from build123d import *

# Parameters (mm, degrees)
SKETCH1_R           = 1.524
BOSS_EXTRUDE1_DEPTH = 6.35


with BuildPart() as part:
    # Sketch1 → Boss-Extrude1 (new body)
    with BuildSketch(Plane(origin=(0, 0, 0), x_dir=(1, 0, 0), z_dir=(0, 1, 0))):
        with BuildLine():
            Line((23.368, 0), (17.018, 0))
            Line((17.018, 0), (17.018, 5.534999979))
            Line((17.018, 5.534999979), (19.058999982, 5.534999979))
            Line((19.058999982, 5.534999979), (19.058999982, 8.435000021))
            Line((19.058999982, 8.435000021), (17.018, 8.435000021))
            Line((17.018, 8.435000021), (17.018, 13.97))
            Line((17.018, 13.97), (12.7, 13.97))
            Line((12.7, 13.97), (12.7, 8.435000021))
            Line((12.7, 8.435000021), (10.659000018, 8.435000021))
            Line((10.659000018, 8.435000021), (10.659000018, 5.534999979))
            Line((10.659000018, 5.534999979), (12.7, 5.534999979))
            Line((12.7, 5.534999979), (12.7, 0))
            Line((12.7, 0), (6.35, 0))
            Line((6.35, 0), (6.35, -6.35))
            Line((6.35, -6.35), (0, -6.35))
            Line((0, -6.35), (0, 0))
            Line((0, 0), (-15.24, 22.286579861))
            ThreePointArc((-15.24, 22.286579861), (-12.038790491, 39.334629649), (5.009259297, 36.133420139))
            Line((5.009259297, 36.133420139), (29.718, 0))
            Line((29.718, 0), (29.718, -6.35))
            Line((29.718, -6.35), (23.368, -6.35))
            Line((23.368, -6.35), (23.368, 0))
        make_face()
        with Locations(Location((-5.115370351, 29.21, 0), (0, 0, 270))):
            Circle(SKETCH1_R, mode=Mode.SUBTRACT)
    extrude(amount=BOSS_EXTRUDE1_DEPTH)


solid = part.part
Verification items for the finished model (mm, model axes). A direction names the side the tool comes from. Round coordinates to 2 decimals unless told otherwise and drop trailing zeros. Loops run counter-clockwise (first coordinate to the right, second up) from the corner with the lowest first, then second, coordinate; pieces in that order, holes last. Notation, with made-up numbers: (80.25, -31.75) - (106.25, -31.75) arc R13 cw to (106.25, -14.75) - close; hole circle Ø11 at (66.25, 17.5). An arc over 180 degrees is marked (long way). Answer in a Markdown table with one row per item. Add a question column.
Q1. Tool access check on faces 1 (the face through (27, 3, 6.35)), 2 (the face through (12, 3, -8.435)), 3 (the face through (15, 3, -13.97)). Record the directions out of +Z, -Z, +X, -X, +Y, -Y that give a thin tool (end or side, any length) a straight path to the whole face; none if there is none.
Q2. Release check for a two-part mould opening along X. For faces 4 (the face through (10, 3, 0)), 5 (the face through (29.718, 3, 3)), 6 (the face through (0, 3, 3)), 7 (the face through (12.7, 3, -11)) record: pulls with the +X half, pulls with the -X half, needs draft (parallel to the pull), parting line crosses it, or undercut.
Q3. Material ranges on line 1 (X direction, y = 5.5, z = -29.5); line 2 (X direction, y = 3.75, z = -8.5); line 3 (X direction, y = 5.5, z = -21), recorded low to high.
Q4. Gauge pin test, flat ends, axial feed: pin 1 (0.6 mm diameter, centred on x = 18, y = 3, fed in from +Z); pin 2 (2 mm diameter, centred on x = 0.5, z = -9.5, fed in from -Y); pin 3 (1.7 mm diameter, centred on y = 2, z = -11.5, fed in from +X); pin 4 (2.5 mm diameter, centred on y = 4.5, z = -7, fed in from -X). Record the tip position at first contact, or that the pin passes through.
Q5. Section check D-D on x = 7.5. Enter the section's corners in (y, z), plus the area to 3 significant figures.
Q6. Section check B-B on y = 5.25. Enter the section's corners in (x, z) (3 decimals), plus the area to 3 significant figures.
Q7. Section check C-C on z = -34. Enter the section's corners in (x, y), plus the area to 3 significant figures.
Q8. Section check A-A on z = -29.21. Enter the section's corners in (x, y).
Found:
| question | item | result |
|---|---|---|
| 1 | face 1 | +Z, +X, -X, +Y, -Y |
| 1 | face 2 | +Y, -Y |
| 1 | face 3 | +Z, +Y, -Y |
| 2 | face 4 | undercut |
| 2 | face 5 | pulls with the +X half |
| 2 | face 6 | pulls with the -X half |
| 2 | face 7 | undercut |
| 3 | line 1 | x = -17.38 to -6.61, -3.62 to 9.55 |
| 3 | line 2 | x = -5.81 to 12.7, 17.02 to 23.91 |
| 3 | line 3 | x = -14.36 to 15.36 |
| 4 | pin 1 | stops at z = 0 |
| 4 | pin 2 | stops at y = 0 |
| 4 | pin 3 | stops at x = 22.44 |
| 4 | pin 4 | stops at x = -5.64 |
| 5 | outline | (0, -32.49) - (6.35, -32.49) - (6.35, 0) - (0, 0) - close |
| 5 | area | 206 mm² |
| 6 | outline | (-15.24, -22.287) arc R12.265 ccw to (5.009, -36.133) - (29.718, 0) - (29.718, 6.35) - (23.368, 6.35) - (23.368, 0) - (17.018, 0) - (17.018, -5.535) - (19.059, -5.535) - (19.059, -8.435) - (17.018, -8.435) - (17.018, -13.97) - (12.7, -13.97) - (12.7, -8.435) - (10.659, -8.435) - (10.659, -5.535) - (12.7, -5.535) - (12.7, 0) - (6.35, 0) - (6.35, 6.35) - (0, 6.35) - (0, 0) - close; hole circle Ø3.048 at (-5.115, -29.21) |
| 6 | area | 1,110 mm² |
| 7 | outline | (-16.41, 0) - (6.47, 0) - (6.47, 6.35) - (-16.41, 6.35) - close |
| 7 | area | 145 mm² |
| 8 | outline | (-17.38, 0) - (-6.64, 0) - (-6.64, 6.35) - (-17.38, 6.35) - close; (-3.59, 0) - (9.74, 0) - (9.74, 6.35) - (-3.59, 6.35) - close |
